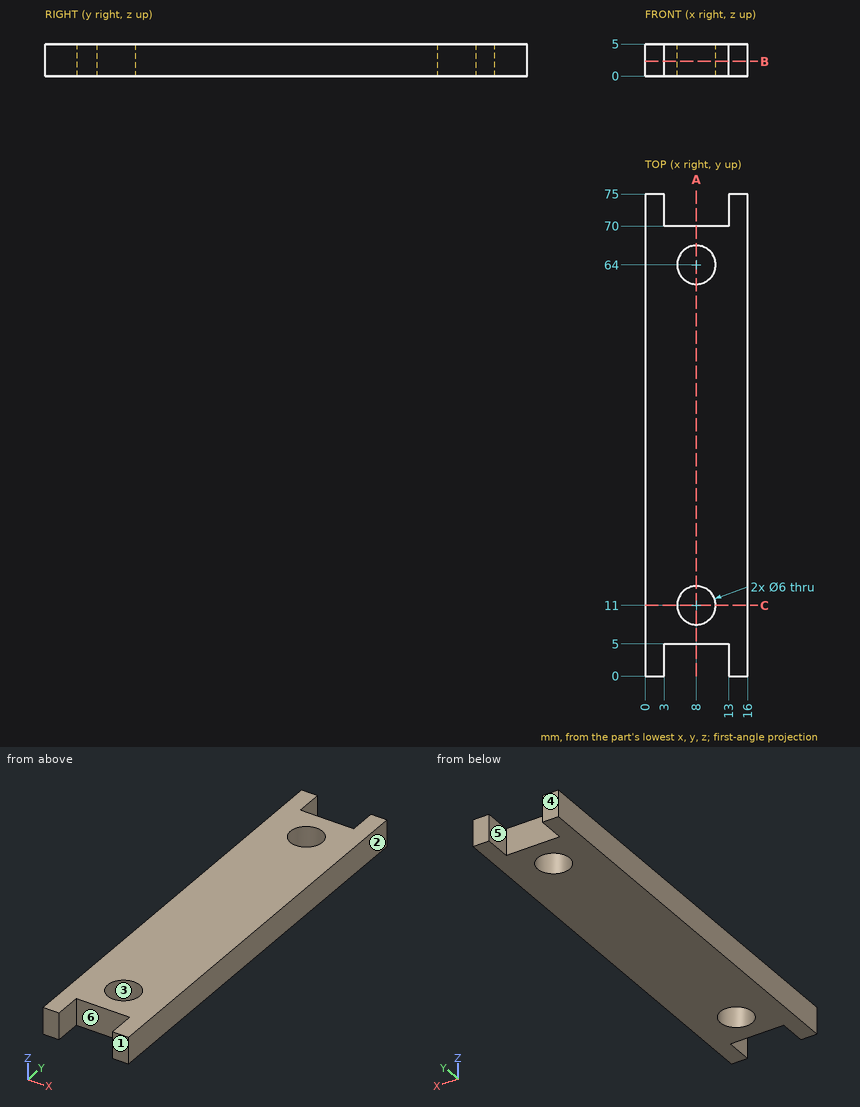
Here's the drawing with two shaded views (mm, measured from the low corner). I have some questions. A direction names the side the tool comes from. Coordinates: 2 decimals unless noted, no trailing zeros. Write each loop counter-clockwise with the first axis right and the second up, starting at its lowest first coordinate (ties: lowest second). Pieces come first, ordered by that corner, then holes. Notation, with made-up numbers: M 29,-40 L 63,-40 A15 cw 63,-34 Z; hole C 24.25,58 d6. An arc over 180 degrees is marked long. Answer as CSV lines item,"result".
Item 1: Please list where these lines run through material, in increasing order: line 1 along Y through (x, z) = (8, 1.8); line 2 along X through (y, z) = (11, 1.5); line 3 along Y through (x, z) = (4.25, 4.3).
Geometry results:
line 1,"y = 5 to 8, 14 to 61, 67 to 70"
line 2,"x = 0 to 5, 11 to 16"
line 3,"y = 5 to 70"
Item 2: Imagine slicing it at B-B on z = 2.3. List the corners of the cut face in (x, y) for me.
Geometry results:
outline,"M 0,0 L 3,0 L 3,5 L 13,5 L 13,0 L 16,0 L 16,75 L 13,75 L 13,70 L 3,70 L 3,75 L 0,75 Z; hole C 8,11 d6; hole C 8,64 d6"
Item 3: Imagine slicing it at A-A on x = 8. List the corners of the cut face in (y, z) for me.
Geometry results:
outline,"M 5,0 L 8,0 L 8,5 L 5,5 Z; M 14,0 L 61,0 L 61,5 L 14,5 Z; M 67,0 L 70,0 L 70,5 L 67,5 Z"
Item 4: On a 3-axis mill with a long thin cutter (end or side, diameter ignored), from which of +Z, -Z, +X, -X, +Y, -Y can I reach the whole of each face in a straight line? I mean the marked faces 4, 5 and 6. Say none if no direction works.
Geometry results:
face 4,"+Z, -Z, +X, -X, +Y"
face 5,"+Z, -Z, +Y"
face 6,"+Z, -Z, -Y"
Item 5: We'd pull the mould along Y, two halves only. Please class the marked faces 1, 2 and 3: +Y half, -Y half, draft (parallel to the pull), parting line (faces both ways), or undercut.
Geometry results:
face 1,"-Y half"
face 2,"draft"
face 3,"undercut"
Item 6: Imagine slicing it at C-C on y = 11. List the corners of the cut face in (x, z) for me, plus the area to 3 significant figures.
Geometry results:
outline,"M 0,0 L 5,0 L 5,5 L 0,5 Z; M 11,0 L 16,0 L 16,5 L 11,5 Z"
area,"50.0 mm2"
Item 7: I'm going to push flat-ended pins straight in: P1, Ø1.5, axis at x = 9.5, z = 3.5, coming from the +Y side; P2, Ø2.5, axis at x = 8.5, z = 1.5, coming from the -Y side. Where does each tip first touch, or does it pass through?
Geometry results:
P1,"stops at y = 70"
P2,"stops at y = 5"
